Can you work these out from the model? Positions are in its coordinate system, mm. A direction names the side the tool comes from. Give positions to 0.01 mm unless a question says otherwise; leave off trailing zeros. Order: outer loops, then holes, each group sorted by start corner. A loop starts at its lowest first (then second) coordinate and runs counter-clockwise, first axis right, second up. Notation, with made-up numbers: M 67.5,-1.75 L 107.5,-1.75 A23 cw 107.5,17.25 Z; hole C 78,56.25 d1. An arc over 180 degrees is marked long. Use a Markdown table: item, result. Add a question column.
from build123d import *

# Parameters (mm, degrees)
F1_DEPTH = 6.35
F2_R     = 44.44999


# Not quite as in the source:
# - a fillet or chamfer is up to 0.001 mm smaller than in the source, because OpenCascade refuses the exact size


with BuildPart() as f1:
    # F0 (on Top) → F1 (new body)
    with BuildSketch(Plane.XY):
        Polygon((41.275, -44.45), (41.275, 44.45), (-41.275, 44.45), (-41.275, 38.1), (-34.925, 38.1), (-34.925, -38.1), (-41.275, -38.1), (-41.275, -44.45), align=None)
        with BuildLine():
            Line((0, -38.1), (-22.225, -38.1))
            Line((-22.225, -38.1), (-22.225, 38.1))
            Line((-22.225, 38.1), (0, 38.1))
            ThreePointArc((0, 38.1), (38.1, 0), (0, -38.1))
        make_face(mode=Mode.SUBTRACT)
    extrude(amount=F1_DEPTH)

    # F2 (radius 44.45 in the source; OpenCascade refuses exactly that, so slightly less here)
    f2_edges = [f1.edges().sort_by_distance(p)[0] for p in [
        (41.275, -44.45, 3.175),
        (41.275, 44.45, 3.175),
    ]]
    fillet(f2_edges, radius=F2_R)


solid = f1.part
1. I need wall thicknesses on L1, parallel to Y at x = -6, z = 4.25; L2, parallel to Y at x = -1, z = 6; L3, parallel to X at y = -7, z = 4 (3 decimals). Which ranges of each line are inside material? Lowest first, please. Write a range as [from, to].
2. On a 3-axis mill with a long thin cutter (end or side, diameter ignored), from which of +Z, -Z, +X, -X, +Y, -Y can I reach the whole of each face in a straight line? I mean faces 4 (the face through (-38, 38.1, 3)), 5 (the face through (-22, 44.45, 3)), 6 (the face through (38.09, 0.84, 3.13)). Say none if no direction works.
3. We'd pull the mould along X, two halves only. Please class faces 1 (the face through (28.6, -31.083, 3.219)), 2 (the face through (-11, -38.1, 3)), 3 (the face through (-38, -38.1, 3)): +X half, -X half, draft (parallel to the pull), parting line (faces both ways), or undercut.
4. If we section it at C-C, the plane y = -15: List the corners of the cut face in (x, z) for me (3 decimals), then the cut area to 3 significant figures.
5. If we section it at A-A, the plane x = -19: List the corners of the cut face in (y, z) for me.
6. Will these pins go through, and if not, where does the flat tip stop? pin 1 (1 mm diameter, centred on y = 29.5, z = 4, fed in from +X); pin 2 (3 mm diameter, centred on y = 10, z = 0.5, fed in from +X); pin 3 (3 mm diameter, centred on y = -14, z = 4.5, fed in from +X).
Geometry results:
| question | item | result |
|---|---|---|
| 1 | L1 | y = [-44.45, -38.1], [38.1, 44.45] |
| 1 | L2 | y = [-44.4, -38.1], [38.1, 44.4] |
| 1 | L3 | x = [-34.925, -22.225], [37.451, 40.72] |
| 2 | face 4 | +Z, -Z, -X |
| 2 | face 5 | +Z, -Z, +X, -X, +Y |
| 2 | face 6 | +Z, -Z |
| 3 | face 1 | +X half |
| 3 | face 2 | undercut |
| 3 | face 3 | draft |
| 4 | outline | M -34.925,0 L -22.225,0 L -22.225,6.35 L -34.925,6.35 Z; M 35.023,0 L 38.668,0 L 38.668,6.35 L 35.023,6.35 Z |
| 4 | area | 104 mm^2 |
| 5 | outline | M -44.45,0 L -38.1,0 L -38.1,6.35 L -44.45,6.35 Z; M 38.1,0 L 44.45,0 L 44.45,6.35 L 38.1,6.35 Z |
| 6 | pin 1 | stops at x = 30.51 |
| 6 | pin 2 | stops at x = 40.45 |
| 6 | pin 3 | stops at x = 39.48 |
